Can you work these out from the model? Positions are in its coordinate system, mm. Coordinates: 2 decimals unless noted, no trailing zeros. Order: outer loops, then holes, each group sorted by start corner. A loop starts at its lowest first (then second) coordinate and runs counter-clockwise, first axis right, second up. Notation, with made-up numbers: (42.5, -26.75) - (98.5, -26.75) arc R20 cw to (98.5, 1.25) - close; hole circle Ø11 at (36, -13). An arc over 180 degrees is marked (long way). Use a Markdown table: item, result. Add a question column.
(1) If I drill on L1, parallel to X at y = -2, z = 31 (3 decimals); L2, parallel to X at y = 8.5, z = -18 (3 decimals); L3, parallel to X at y = 22.5, z = -5, over which ranges is the centre line in solid material (lowest first)? Write a range as [from, to].
(2) I want a section at A-A (z = -1). List the corners of the cut face in (x, y) for me (3 decimals), and give its area (3 significant figures).
(3) I want a section at B-B (y = 0). List the corners of the cut face in (x, z) for me (3 decimals), and give its area (3 significant figures).
```python
from build123d import *

# Parameters (mm, degrees)
F0_W     = 50.8
F0_H     = 101.6
F1_DEPTH = 762
F2_W     = 25.4
F2_H     = 44.45
F3_DEPTH = 50.801
F4_W     = 44.45
F4_H     = 25.4
F5_DEPTH = 101.601


# Not quite as in the source:
# - a pattern or mirror of a feature is missing from the dataset's text; its kind, count and spacing are read off the source's solid


with BuildPart() as f1:
    # F0 (on Right) → F1 (new body, symmetric)
    with BuildSketch(Plane.YZ):
        Rectangle(F0_W, F0_H)
    extrude(amount=F1_DEPTH, both=True)

    # F2 (on face) → F3 (cut, through all)
    with BuildSketch(Plane(origin=(0, 25.4, 0), x_dir=(-1, 0, 0), z_dir=(0, 1, 0))):
        Rectangle(F2_W, F2_H)
    extrude(amount=-F3_DEPTH, mode=Mode.SUBTRACT)

    # F4 (on face) → F5 (cut, through all)
    with BuildSketch(Plane.XY.offset(50.8)):
        with Locations((-609.6, 0)):
            Rectangle(F4_W, F4_H)
    f5 = extrude(amount=-F5_DEPTH, mode=Mode.SUBTRACT)

    # F5_copies: F5 across plane
    add(f5.mirror(Plane(origin=(0, 0, 0), x_dir=(0, 0, 1), z_dir=(1, 0, 0))), mode=Mode.SUBTRACT)


solid = f1.part
```
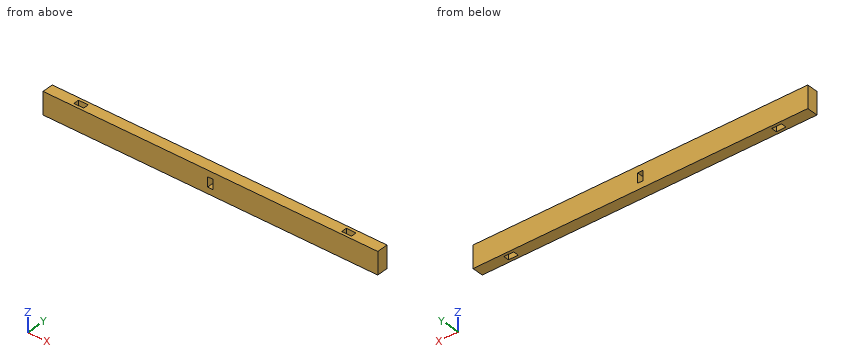
Answers follow:
| question | item | result |
|---|---|---|
| 1 | L1 | x = [-762, -631.825], [-587.375, 587.375], [631.825, 762] |
| 1 | L2 | x = [-762, -631.825], [-587.375, -12.7], [12.7, 587.375], [631.825, 762] |
| 1 | L3 | x = [-762, -12.7], [12.7, 762] |
| 2 | outline | (-762, -25.4) - (-12.7, -25.4) - (-12.7, 25.4) - (-762, 25.4) - close; (12.7, -25.4) - (762, -25.4) - (762, 25.4) - (12.7, 25.4) - close; hole (-631.825, -12.7) - (-587.375, -12.7) - (-587.375, 12.7) - (-631.825, 12.7) - close; hole (587.375, -12.7) - (631.825, -12.7) - (631.825, 12.7) - (587.375, 12.7) - close |
| 2 | area | 73,900 mm² |
| 3 | outline | (-762, -50.8) - (-631.825, -50.8) - (-631.825, 50.8) - (-762, 50.8) - close; (-587.375, -50.8) - (587.375, -50.8) - (587.375, 50.8) - (-587.375, 50.8) - close; (631.825, -50.8) - (762, -50.8) - (762, 50.8) - (631.825, 50.8) - close; hole (-12.7, -22.225) - (12.7, -22.225) - (12.7, 22.225) - (-12.7, 22.225) - close |
| 3 | area | 145,000 mm² |
